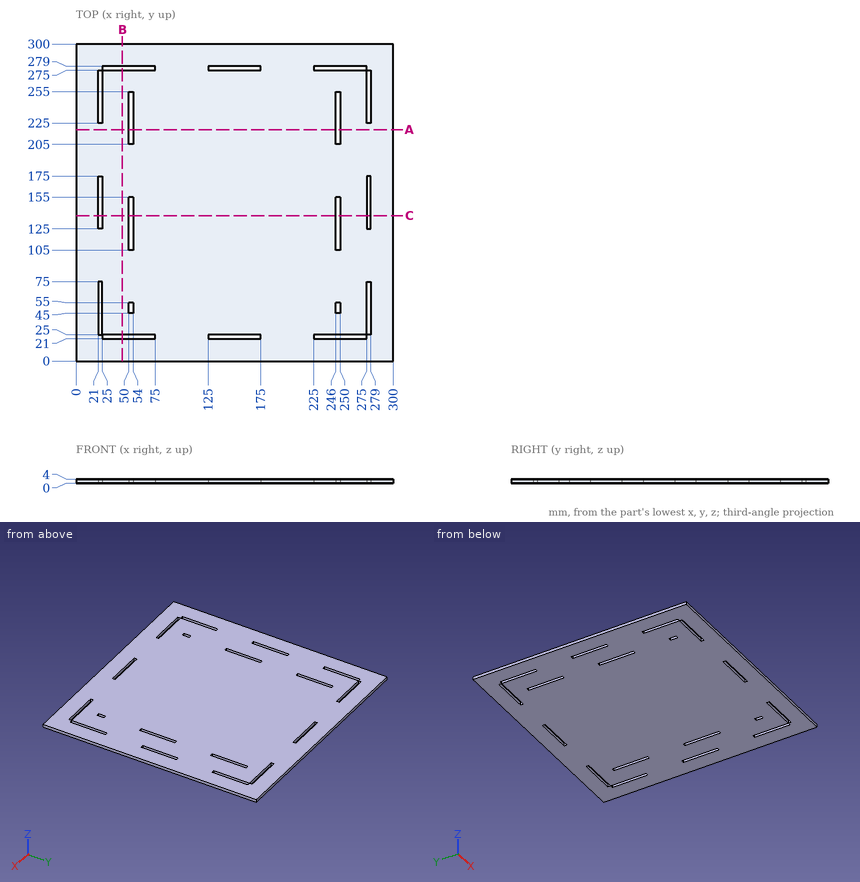
Input: dimensioned drawing with shaded views. Units: mm. Origin: part minimum x, y, z. Round coordinates to 2 decimals unless told otherwise and drop trailing zeros. Loops run counter-clockwise (first coordinate to the right, second up) from the corner with the lowest first, then second, coordinate; pieces in that order, holes last.
1) Material intervals for line 1 (X direction, y = 172, z = 2.45); line 2 (X direction, y = 148.5, z = 3.7), sorted ascending.
Ans:
line 1: x = 0 to 21, 25 to 275, 279 to 300
line 2: x = 0 to 21, 25 to 50, 54 to 246, 250 to 275, 279 to 300
2) Section query C-C on y = 137.5. Return the cut outline in (x, z), plus the area to 3 significant figures.
Ans:
outline: (0, 0) - (21, 0) - (21, 4) - (0, 4) - close; (25, 0) - (50, 0) - (50, 4) - (25, 4) - close; (54, 0) - (246, 0) - (246, 4) - (54, 4) - close; (250, 0) - (275, 0) - (275, 4) - (250, 4) - close; (279, 0) - (300, 0) - (300, 4) - (279, 4) - close
area: 1,140 mm2
3) Section query B-B on x = 44. Return the cut outline in (y, z).
Ans:
outline: (0, 0) - (21, 0) - (21, 4) - (0, 4) - close; (25, 0) - (275, 0) - (275, 4) - (25, 4) - close; (279, 0) - (300, 0) - (300, 4) - (279, 4) - close
4) Section query A-A on y = 219. Return the cut outline in (x, z), plus the area to 3 significant figures.
Ans:
outline: (0, 0) - (50, 0) - (50, 4) - (0, 4) - close; (54, 0) - (246, 0) - (246, 4) - (54, 4) - close; (250, 0) - (300, 0) - (300, 4) - (250, 4) - close
area: 1,170 mm2
